Source: CAD feature listing. Evaluate the final solid. Frame: model axes, mm. Round coordinates to 2 decimals unless told otherwise and drop trailing zeros. Order: outer loops, then holes, each group sorted by start corner. A loop starts at its lowest first (then second) coordinate and runs counter-clockwise, first axis right, second up. Notation, with made-up numbers: M 55,-37 L 74,-37 A14 cw 74,-14 Z; hole C 17.25,87.5 d11. An arc over 180 degrees is marked long. Use one line per item in the form item = value. Start each with the question number.
Q1. Section C-C (z = 21.5). Return the cut outline in (x, y), plus the area to 3 significant figures.
Q2. Section A-A (y = 12). Return the cut outline in (x, z).
Q3. Section B-B (x = 15). Return the cut outline in (y, z), plus the area to 3 significant figures.
Q4. Material intervals for probe 1 along Z at (x, y) = (6.5, -17); probe 2 along Z at (x, y) = (22, 1); probe 3 along X at (y, z) = (-4, 17.5), sorted ascending.
from build123d import *

# Parameters (mm, degrees)
F0_R     = 12.7
F1_DEPTH = 25.4


# Not quite as in the source:
# - the program builds the solid bodies; features that only make, move or delete a surface that nothing else refers to are left out


with BuildPart() as f1:
    # F0 (on Front) → F1 (new body, symmetric)
    with BuildSketch(Plane.XZ):
        Polygon((-38.1, 25.4), (-38.1, -25.4), (38.1, -25.4), (38.1, 0), (0, 25.4), align=None)
        Circle(F0_R, mode=Mode.SUBTRACT)
        Circle(F0_R)
    extrude(amount=F1_DEPTH, both=True)


solid = f1.part
Results list:
q1.outline = M -38.1,-25.4 L 5.85,-25.4 L 5.85,25.4 L -38.1,25.4 Z
q1.area = 2,230 mm2
q2.outline = M -38.1,-25.4 L 38.1,-25.4 L 38.1,0 L 0,25.4 L -38.1,25.4 Z
q3.outline = M -25.4,-25.4 L 25.4,-25.4 L 25.4,15.4 L -25.4,15.4 Z
q3.area = 2,070 mm2
q4.probe_1 = -25.4 to 21.07
q4.probe_2 = -25.4 to 10.73
q4.probe_3 = -38.1 to 11.85
